```python
from build123d import *

# Parameters (mm, degrees)
F0_W     = 300
F0_H     = 150
F1_DEPTH = 327
F2_T     = -2.5
F4_DEPTH = 346


with BuildPart() as f1:
    # F0 (on Top) → F1 (new body)
    with BuildSketch(Plane.XY):
        with Locations((150, 75)):
            Rectangle(F0_W, F0_H)
    extrude(amount=F1_DEPTH)

    # F2
    f2_openings = [f1.faces().sort_by_distance(p)[0] for p in [
        (150, 75, 327),
    ]]
    offset(amount=F2_T, openings=f2_openings)

    # F3 (on face) → F4 (cut)
    with BuildSketch(Plane.YZ.offset(300)):
        Polygon((0, 295.443952), (150, 327), (0, 327), align=None)
    extrude(amount=-F4_DEPTH, mode=Mode.SUBTRACT)


solid = f1.part
```
Design review of the part built by this model. Coordinates are the model's own, in mm. A direction names the side the tool comes from. Coordinates: 2 decimals unless noted, no trailing zeros. Order: outer loops, then holes, each group sorted by start corner. A loop starts at its lowest first (then second) coordinate and runs counter-clockwise, first axis right, second up. Notation, with made-up numbers: (13.25, -25) - (26.25, -25) arc R6 ccw to (26.25, -15) - close; hole circle Ø8 at (9.25, -25.5). An arc over 180 degrees is marked (long way). One line per question, with ' | ' between items.
Q1. Consider section B-B, the plane x = 128.5. Give the boundary of the cut face in (y, z), then the cut area to 3 significant figures.
Answer key:
outline: (0, 0) - (150, 0) - (150, 327) - (147.5, 326.47) - (147.5, 2.5) - (2.5, 2.5) - (2.5, 295.97) - (0, 295.44) - close | area: 1,920 mm2
Q2. For faces 4 (the flat face through (0, 74, 161)), 5 (the flat face through (148, 147.5, 162)), list the 3-axis set-ups (+Z, -Z, +X, -X, +Y, -Y) from which the entire face can be reached by the end or side of a thin tool; tool diameter is ignored.
Answer key:
face 4: +Z, -Z, -X, +Y, -Y | face 5: +Z
Q3. The part is to be moulded in two halves that separate along Y. For faces 1 (the flat face through (148, 0, 146)), 2 (the flat face through (148, 2.5, 147)), 3 (the flat face through (148, 150, 161)), say which applies: +Y half, -Y half, draft (parallel to the pull), parting line (faces both ways), or undercut.
Answer key:
face 1: -Y half | face 2: undercut | face 3: +Y half
Q4. Consider section A-A, the plane z = 115.5. Give the boundary of the cut face in (x, y).
Answer key:
outline: (0, 0) - (300, 0) - (300, 150) - (0, 150) - close; hole (2.5, 2.5) - (297.5, 2.5) - (297.5, 147.5) - (2.5, 147.5) - close
Q5. Consider section C-C, the plane y = 88.5. Give the boundary of the cut face in (x, z).
Answer key:
outline: (0, 0) - (300, 0) - (300, 314.06) - (297.5, 314.06) - (297.5, 2.5) - (2.5, 2.5) - (2.5, 314.06) - (0, 314.06) - close
Q6. To check wall thickness, follow line 1 along X through (y, z) = (114.5, 61); line 2 along Y through (x, z) = (283.5, 125); line 3 along Z through (x, y) = (25, 58). State the ranges of each line that lie inside material, in increasing order.
Answer key:
line 1: x = 0 to 2.5, 297.5 to 300 | line 2: y = 0 to 2.5, 147.5 to 150 | line 3: z = 0 to 2.5
Q7. Clearance check with a flat-ended pin moving along its axis: pin 1 Ø5 at (x, y) = (177.5, 17.5) entering from +Z. State where the tip first meets the part, or that it passes through.
Answer key:
pin 1: stops at z = 2.5
